The figure shows three views and two pictorial views of one solid part (mm, origin at its lowest corner). Answer the questions. A direction names the side the tool comes from. Give positions to 0.01 mm unless a question says otherwise; leave off trailing zeros. Loops run counter-clockwise (first coordinate to the right, second up) from the corner with the lowest first, then second, coordinate; pieces in that order, holes last. Notation, with made-up numbers: (-33, 15) -> (26, 15) arc R26 ccw to (26, 47) -> close; hole circle Ø7 at (-21, 3). An arc over 180 degrees is marked (long way). Answer as CSV lines item,"result". Start each with the question number.
1. Find section C-C, the plane z = 0.3. Count the separate pieces of the cut face and the enclosed holes in it.
2. A tool of negligible diameter and unlimited length cuts with its end or side. For the marked faces 4, 5 and 6, from which of +Z, -Z, +X, -X, +Y, -Y can it reach the whole face along a straight path? Write none if from no direction.
3. Find section D-D, the plane x = 7.5. Give the vertices of the cut face in (y, z) (1 decimal).
4. Find the intervals of material crossed by line 1 along X through (y, z) = (9.75, 0.25); line 2 along Y through (x, z) = (7.5, 2.5) (1 decimal); line 3 along Z through (x, y) = (9, 10), in increasing order.
5. Determine the mould class of the marked faces 1, 2 and 3 for opening direction X: +X half, -X half, draft (parallel to the pull), parting line (faces both ways), or undercut.
6. Flat-ended cylindrical pins translate along their axes: pin 1 Ø4.5 at (x, y) = (8.5, 8.5) entering from +Z; pin 2 Ø1.5 at (x, z) = (3, 4) entering from +Y; pin 3 Ø0.9 at (y, z) = (8.5, 2) entering from -X. Find the tip coordinate at first contact, or state that the pin passes through.
7. Find section B-B, the plane y = 11. Give the vertices of the cut face in (x, z), and give its area (3 significant figures).
8. Find section A-A, the plane y = 2.5. Give the vertices of the cut face in (x, z) (1 decimal).
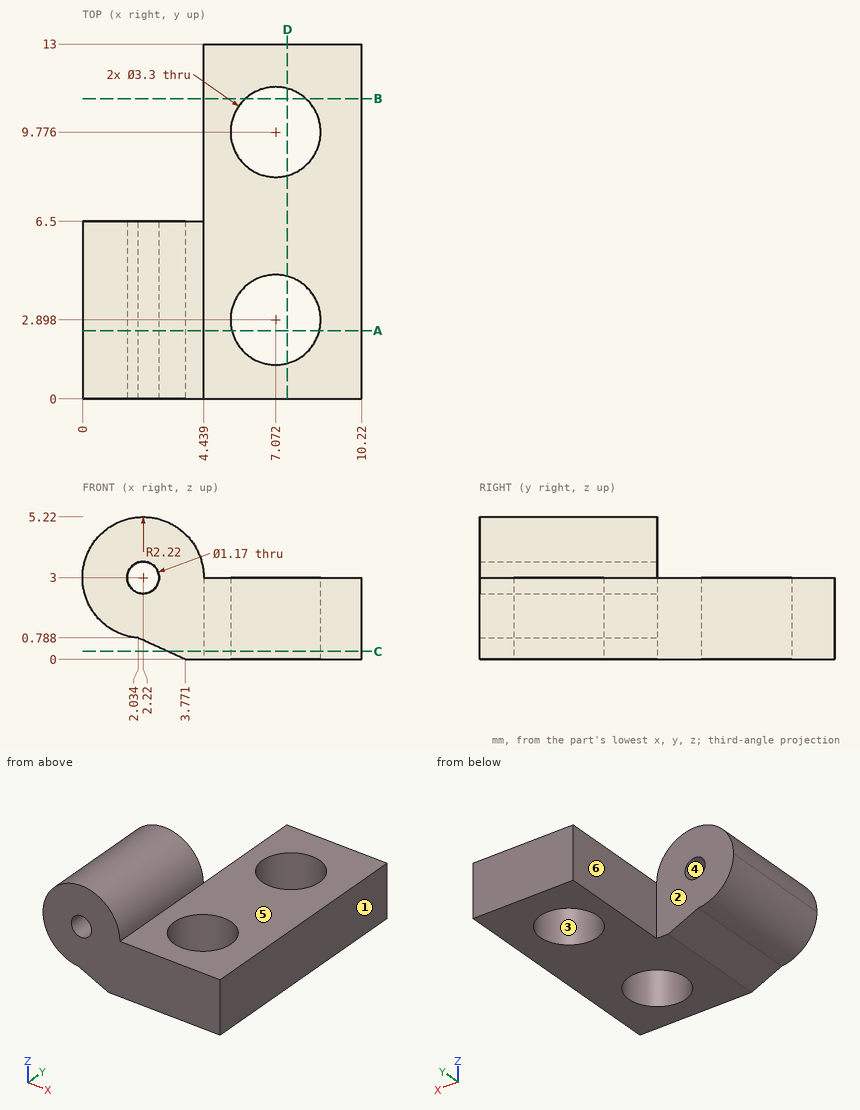
Resolved:
1,separate pieces,"1"
1,enclosed holes,"2"
2,face 4,"+Y, -Y"
2,face 5,"+Z, +X, +Y, -Y"
2,face 6,"+Z, -Z, -X, +Y"
3,outline,"(0, 0) -> (1.3, 0) -> (1.3, 3) -> (0, 3) -> close; (4.5, 0) -> (8.2, 0) -> (8.2, 3) -> (4.5, 3) -> close; (11.4, 0) -> (13, 0) -> (13, 3) -> (11.4, 3) -> close"
4,line 1,"x = 4.44 to 5.42, 8.72 to 10.22"
4,line 2,"y = 0 to 1.3, 4.5 to 8.2, 11.4 to 13"
4,line 3,"z = 0 to 3"
5,face 1,"+X half"
5,face 2,"draft"
5,face 3,"undercut"
6,pin 1,"stops at z = 3"
6,pin 2,"stops at y = 6.5"
6,pin 3,"stops at x = 4.44"
7,outline,"(4.44, 0) -> (5.97, 0) -> (5.97, 3) -> (4.44, 3) -> close; (8.18, 0) -> (10.22, 0) -> (10.22, 3) -> (8.18, 3) -> close"
7,area,"10.7 mm^2"
8,outline,"(2, 0.8) -> (3.8, 0) -> (5.5, 0) -> (5.5, 3) -> (4.4, 3) arc R2.2 ccw (long way) to start; (8.7, 0) -> (10.2, 0) -> (10.2, 3) -> (8.7, 3) -> close; hole circle Ø1.2 at (2.2, 3)"
